Could you check a few things on this model? Use its own coordinates, in mm. Give positions to 0.01 mm unless a question says otherwise; leave off trailing zeros. Write each loop counter-clockwise with the first axis right and the second up, starting at its lowest first coordinate (ties: lowest second). Pieces come first, ordered by that corner, then holes. Notation, with made-up numbers: M 5,33 L 44,33 A6 ccw 44,41 Z; hole C 76,-19.75 d1. An arc over 180 degrees is marked long. Write each question's results on one line, items separated by ' | '. Start each with the question number.
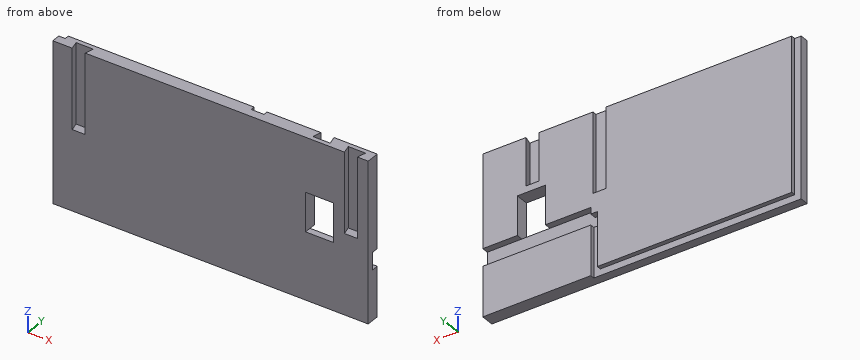
from build123d import *

# Parameters (mm, degrees)
F0_W      = 146
F0_H      = 74
F1_DEPTH  = 6
F2_W      = 13
F2_H      = 18
F3_DEPTH  = 6
F5_DEPTH  = 2
F7_DEPTH  = 3
F6_W      = 6
F6_H      = 37
F8_DEPTH  = 2
F10_DEPTH = 37
F11_DEPTH = 37
F12_DEPTH = 22


with BuildPart() as f1:
    # F0 (on Front) → F1 (new body)
    with BuildSketch(Plane.XZ):
        with Locations((73, 37)):
            Rectangle(F0_W, F0_H)
    extrude(amount=F1_DEPTH)

    # F2 (on face) → F3 (cut)
    with BuildSketch(Plane.XZ.offset(6)):
        with Locations((123.5, 40)):
            Rectangle(F2_W, F2_H)
    extrude(amount=-F3_DEPTH, mode=Mode.SUBTRACT)

    # F4 (on face) → F5 (cut)
    with BuildSketch(Plane(origin=(0, 0, 0), x_dir=(-1, 0, 0), z_dir=(0, 1, 0))):
        Polygon((-96, 23), (-96, 0), (0, 0), (0, 74), (-3, 74), (-3, 3), (-93, 3), (-93, 23), align=None)
    extrude(amount=-F5_DEPTH, mode=Mode.SUBTRACT)

    # F6 (on face) → F7 (cut)
    with BuildSketch(Plane(origin=(0, 0, 0), x_dir=(-1, 0, 0), z_dir=(0, 1, 0))):
        Polygon((-146, 31), (-146, 23), (-96, 23), (-93, 23), (-93, 28), (-96, 28), (-96, 31), (-117, 31), (-130, 31), align=None)
    extrude(amount=-F7_DEPTH, mode=Mode.SUBTRACT)

    # F6 (on face) → F8 (cut)
    with BuildSketch(Plane(origin=(0, 0, 0), x_dir=(-1, 0, 0), z_dir=(0, 1, 0))):
        with Locations((-92, 55.5)):
            Rectangle(F6_W, F6_H)
    extrude(amount=-F8_DEPTH, mode=Mode.SUBTRACT)

    # F9 (on face) → F10 (cut)
    with BuildSketch(Plane.XY.offset(74)):
        Polygon((141, -6), (142, -2), (134, -2), (135, -6), align=None)
    extrude(amount=-F10_DEPTH, mode=Mode.SUBTRACT)

    # F9 (on face) → F11 (cut)
    with BuildSketch(Plane.XY.offset(74)):
        Polygon((15, -6), (16, -2), (8, -2), (9, -6), align=None)
    extrude(amount=-F11_DEPTH, mode=Mode.SUBTRACT)

    # F9 (on face) → F12 (cut)
    with BuildSketch(Plane.XY.offset(74)):
        Polygon((126, -4), (127, -4), (126, 0), (120, 0), (119, -4), (120, -4), align=None)
    extrude(amount=-F12_DEPTH, mode=Mode.SUBTRACT)


solid = f1.part
Q1. If we section it at C-C (x = 100): Please give me the cut outline in (y, z).
Q2. Please list where these lines run through material, in increasing order: line 1 (X direction, y = -1.5, z = 41.5); line 2 (Z direction, x = 133.5, y = -2.5); line 3 (X direction, y = -5.35, z = 61). Write a range as [from, to].
Q3. If we section it at A-A (z = 35): Please give me the cut outline in (x, y).
Q4. I'm going to push flat-ended pins straight in: P1, Ø0.6, axis at x = 91, y = -1, coming from the +Z side; P2, Ø0.9, axis at y = -2, z = 29.5, coming from the +X side; P3, Ø0.6, axis at y = -0.5, z = 53, coming from the -X side. Where does each tip first touch, or does it pass through?
Q5. If we section it at B-B (x = 122): Please give me the cut outline in (y, z), plus the area to 3 significant figures.
Q6. If we section it at D-D (z = 45.5): Please give me the cut outline in (x, y).
Determined:
1) outline: M -6,0 L 0,0 L 0,23 L -3,23 L -3,31 L 0,31 L 0,74 L -6,74 Z
2) line 1: x = [3, 89], [95, 117], [130, 146] | line 2: z = [0, 23], [31, 74] | line 3: x = [0, 8.84], [15.16, 134.84], [141.16, 146]
3) outline: M 0,-6 L 117,-6 L 117,0 L 3,0 L 3,-2 L 0,-2 Z; M 130,-6 L 146,-6 L 146,0 L 130,0 Z
4) P1: stops at z = 37 | P2: stops at x = 96 | P3: stops at x = 3
5) outline: M -6,0 L 0,0 L 0,23 L -3,23 L -3,31 L -6,31 Z; M -6,49 L 0,49 L 0,52 L -4,52 L -4,74 L -6,74 Z | area: 224 mm²
6) outline: M 0,-6 L 9,-6 L 8,-2 L 16,-2 L 15,-6 L 117,-6 L 117,0 L 95,0 L 95,-2 L 89,-2 L 89,0 L 3,0 L 3,-2 L 0,-2 Z; M 130,-6 L 135,-6 L 134,-2 L 142,-2 L 141,-6 L 146,-6 L 146,0 L 130,0 Z
